Read the model definition and answer for the solid it produces. Units are mm, in the model's axes. A direction names the side the tool comes from. Coordinates: 2 decimals unless noted, no trailing zeros. Loops run counter-clockwise (first coordinate to the right, second up) from the corner with the lowest first, then second, coordinate; pieces in that order, holes last. Notation, with made-up numbers: M 3.5,88.5 L 53.5,88.5 A18 cw 53.5,105.5 Z; hole C 76,38 d10. An arc over 180 degrees is marked long. Put each result on its own line as item: value.
from build123d import *
from build123d.topology import SkipClean

# Parameters (mm, degrees)
SKETCH1_W           = 65
SKETCH1_H           = 18.4
BOSS_EXTRUDE1_DEPTH = 7.5
SKETCH2_R           = 10
BOSS_EXTRUDE2_DEPTH = 7.5
CUT_EXTRUDE1_DEPTH  = 7.5
BOSS_EXTRUDE3_START = -7.5
BOSS_EXTRUDE3_DEPTH = 7.5
CUT_EXTRUDE2_START  = -7.5
CUT_EXTRUDE2_DEPTH  = 7.5
SKETCH6_R           = 2.0193
CUT_EXTRUDE3_DEPTH  = 7.5
SKETCH11_R          = 3.175
CUT_EXTRUDE6_DEPTH  = 81.999212959
SKETCH1_4_W         = 65
SKETCH1_4_H         = 18.4
BOSS_EXTRUDE6_DEPTH = 6.5
CUT_EXTRUDE7_DEPTH  = 81.999212959
SKETCH13_W          = 80
SKETCH13_H          = 33.4
CUT_EXTRUDE8_DEPTH  = 2
SKETCH14_W          = 80
SKETCH14_H          = 33.4
SKETCH14_W_2        = 65
SKETCH14_H_2        = 18.4
BOSS_EXTRUDE7_DEPTH = 2
CUT_EXTRUDE9_DEPTH  = 81.999212959


with BuildPart() as part:
    # Sketch1 → Boss-Extrude1 (new body)
    with BuildSketch(Plane(origin=(0, 0, 0), x_dir=(1, 0, 0), z_dir=(0, 1, 0))):
        Polygon((0, 25.9), (72.5, 25.9), (72.5, -7.5), (-7.5, -7.5), (-7.5, 25.9), align=None)
        with Locations((32.5, 9.2)):
            Rectangle(SKETCH1_W, SKETCH1_H, mode=Mode.SUBTRACT)
    extrude(amount=BOSS_EXTRUDE1_DEPTH)

    # Sketch2 → Boss-Extrude2 (add)
    with BuildSketch(Plane.XY.offset(7.5)):
        with Locations((32.5, 3.75)):
            Circle(SKETCH2_R)
    extrude(amount=-BOSS_EXTRUDE2_DEPTH)

    # Sketch3 → Cut-Extrude1 (cut)
    with BuildSketch(Plane.XY.offset(7.5)):
        with BuildLine():
            ThreePointArc((38.5, 3.75), (33.646103575, 9.639520065), (26.937851135, 6))
            Line((26.937851135, 6), (38.062148865, 1.5))
            ThreePointArc((38.062148865, 1.5), (38.389520065, 2.603896425), (38.5, 3.75))
        make_face()
        with BuildLine():
            Line((38.062148865, 1.5), (26.937851135, 6))
            ThreePointArc((26.937851135, 6), (30.25, -1.812148865), (38.062148865, 1.5))
        make_face()
    extrude(amount=-CUT_EXTRUDE1_DEPTH, mode=Mode.SUBTRACT)

    # Sketch4 → Boss-Extrude3 (add)
    with BuildSketch(Plane(origin=(0, 0, -25.9), x_dir=(-1, 0, 0), z_dir=(0, 0, -1)).offset(BOSS_EXTRUDE3_START)):
        with BuildLine():
            Line((-23.229751891, 0), (-32.5, 0))
            Line((-32.5, 0), (-41.770248109, 0))
            ThreePointArc((-41.770248109, 0), (-32.5, -6.25), (-23.229751891, 0))
        make_face()
        with BuildLine():
            Line((-41.770248109, 7.5), (-32.5, 7.5))
            Line((-32.5, 7.5), (-23.229751891, 7.5))
            ThreePointArc((-23.229751891, 7.5), (-32.5, 13.75), (-41.770248109, 7.5))
        make_face()
        with BuildLine():
            Line((-23.229751891, 7.5), (-32.5, 7.5))
            Line((-32.5, 7.5), (-32.5, 0))
            Line((-32.5, 0), (-23.229751891, 0))
            ThreePointArc((-23.229751891, 0), (-22.684133225, 1.839827375), (-22.5, 3.75))
            ThreePointArc((-22.5, 3.75), (-22.684133225, 5.660172625), (-23.229751891, 7.5))
        make_face()
        with BuildLine():
            Line((-32.5, 0), (-32.5, 7.5))
            Line((-32.5, 7.5), (-41.770248109, 7.5))
            ThreePointArc((-41.770248109, 7.5), (-42.5, 3.75), (-41.770248109, 0))
            Line((-41.770248109, 0), (-32.5, 0))
        make_face()
    extrude(amount=BOSS_EXTRUDE3_DEPTH)

    # Sketch5 → Cut-Extrude2 (cut)
    with BuildSketch(Plane(origin=(0, 0, -25.9), x_dir=(-1, 0, 0), z_dir=(0, 0, -1)).offset(CUT_EXTRUDE2_START)):
        with BuildLine():
            ThreePointArc((-26.5, 3.75), (-31.353896425, 9.639520065), (-38.062148865, 6))
            Line((-38.062148865, 6), (-26.937851135, 1.5))
            ThreePointArc((-26.937851135, 1.5), (-26.610479935, 2.603896425), (-26.5, 3.75))
        make_face()
        with BuildLine():
            Line((-26.937851135, 1.5), (-38.062148865, 6))
            ThreePointArc((-38.062148865, 6), (-34.75, -1.812148865), (-26.937851135, 1.5))
        make_face()
    extrude(amount=CUT_EXTRUDE2_DEPTH, mode=Mode.SUBTRACT)

    # Sketch6 → Cut-Extrude3 (cut)
    with BuildSketch(Plane(origin=(0, 0, -25.9), x_dir=(-1, 0, 0), z_dir=(0, 0, -1))):
        with Locations((-7.1, 3.75)):
            Circle(SKETCH6_R)
        with Locations((-57.9, 3.75)):
            Circle(SKETCH6_R)
    extrude(amount=-CUT_EXTRUDE3_DEPTH, mode=Mode.SUBTRACT)

    # Sketch11 → Cut-Extrude6 (cut, through all)
    with BuildSketch(Plane(origin=(0, 0, -25.9), x_dir=(-1, 0, 0), z_dir=(0, 0, -1))):
        with Locations((-67.5, 3.75)):
            Circle(SKETCH11_R)
    extrude(amount=-CUT_EXTRUDE6_DEPTH, mode=Mode.SUBTRACT)

    # Sketch1_4 → Boss-Extrude6 (add)
    with BuildSketch(Plane(origin=(0, 0, 0), x_dir=(1, 0, 0), z_dir=(0, 1, 0))):
        Polygon((0, 25.9), (72.5, 25.9), (72.5, -7.5), (-7.5, -7.5), (-7.5, 25.9), align=None)
        with Locations((32.5, 9.2)):
            Rectangle(SKETCH1_4_W, SKETCH1_4_H, mode=Mode.SUBTRACT)
    extrude(amount=-BOSS_EXTRUDE6_DEPTH)

    # Sketch3_4 → Cut-Extrude7 (cut, through all)
    with SkipClean():  # the faces are left unmerged after this step: merging them gives an invalid solid
        with BuildSketch(Plane.XY.offset(7.5)):
            with BuildLine():
                ThreePointArc((38.5, 3.75), (33.646103575, 9.639520065), (26.937851135, 6))
                Line((26.937851135, 6), (38.062148865, 1.5))
                ThreePointArc((38.062148865, 1.5), (38.389520065, 2.603896425), (38.5, 3.75))
            make_face()
            with BuildLine():
                Line((38.062148865, 1.5), (26.937851135, 6))
                ThreePointArc((26.937851135, 6), (30.25, -1.812148865), (38.062148865, 1.5))
            make_face()
        extrude(amount=-CUT_EXTRUDE7_DEPTH, mode=Mode.SUBTRACT)

    # Sketch13 → Cut-Extrude8 (cut)
    with SkipClean():  # the faces are left unmerged after this step: merging them gives an invalid solid
        with BuildSketch(Plane.XZ.offset(6.5)):
            with Locations((32.5, -9.2)):
                Rectangle(SKETCH13_W, SKETCH13_H)
        extrude(amount=-CUT_EXTRUDE8_DEPTH, mode=Mode.SUBTRACT)

    # Sketch14 → Boss-Extrude7 (add)
    with SkipClean():  # the faces are left unmerged after this step: merging them gives an invalid solid
        with BuildSketch(Plane(origin=(0, 7.5, 0), x_dir=(1, 0, 0), z_dir=(0, 1, 0))):
            with Locations((32.5, 9.2)):
                Rectangle(SKETCH14_W, SKETCH14_H)
            with Locations((32.5, 9.2)):
                Rectangle(SKETCH14_W_2, SKETCH14_H_2, mode=Mode.SUBTRACT)
        extrude(amount=BOSS_EXTRUDE7_DEPTH)

    # Sketch3_5 → Cut-Extrude9 (cut, through all)
    with SkipClean():  # the faces are left unmerged after this step: merging them gives an invalid solid
        with BuildSketch(Plane.XY.offset(7.5)):
            with BuildLine():
                ThreePointArc((38.5, 3.75), (33.646103575, 9.639520065), (26.937851135, 6))
                Line((26.937851135, 6), (38.062148865, 1.5))
                ThreePointArc((38.062148865, 1.5), (38.389520065, 2.603896425), (38.5, 3.75))
            make_face()
            with BuildLine():
                Line((38.062148865, 1.5), (26.937851135, 6))
                ThreePointArc((26.937851135, 6), (30.25, -1.812148865), (38.062148865, 1.5))
            make_face()
        extrude(amount=-CUT_EXTRUDE9_DEPTH, mode=Mode.SUBTRACT)


solid = part.part
1) Find section B-B, the plane x = 43.5. Write down the section's boundary in (y, z).
Answer list:
outline: M -4.5,-25.9 L 9.5,-25.9 L 9.5,-18.4 L -4.5,-18.4 Z; M -4.5,0 L 9.5,0 L 9.5,7.5 L -4.5,7.5 Z
2) Straight lines are drawn through the part: line 1 (X direction, y = 4, z = 6); line 2 (X direction, y = -2.75, z = -8); line 3 (X direction, y = 1.5, z = -21). For each, find the intervals that lie inside material, in ascending order. Write a range as [from, to].
Answer list:
line 1: x = [-7.5, 26.51], [38.49, 64.33], [70.67, 72.5]
line 2: x = [-7.5, 0], [65, 72.5]
line 3: x = [-7.5, 26.94], [38.06, 65.26], [69.74, 72.5]
3) Find section D-D, the plane y = 11.75. Write down the section's boundary in (x, z), plus the area to 3 significant figures.
Answer list:
outline: M 26.5,-25.9 L 38.5,-25.9 L 38.5,-18.4 L 26.5,-18.4 Z; M 26.5,0 L 38.5,0 L 38.5,7.5 L 26.5,7.5 Z
area: 180 mm^2
4) Given pin 1 Ø4 at (x, z) = (48.5, -19) entering from +Y; pin 2 Ø5 at (x, y) = (67.5, 3.75) entering from +Z, each flat-ended and moving along its own axis, determine where each tip first touches the part or whether it passes through.
Answer list:
pin 1: stops at y = 9.5
pin 2: passes through
5) Determine the mould class of faces 6 (the cylindrical face through (32.63, 13.75, 3.8)), 7 (the cylindrical face through (5.235, 2.977, -22.202)), 8 (the flat face through (65, -1, -9)) for opening direction Y: released by +Y, released by -Y, zero draft, split by the parting line, or undercut.
Answer list:
face 6: released by +Y
face 7: undercut
face 8: zero draft
6) Find section C-C, the plane z = -16. Write down the section's boundary in (x, y) (3 decimals).
Answer list:
outline: M -7.5,-4.5 L 0,-4.5 L 0,9.5 L -7.5,9.5 Z; M 65,-4.5 L 72.5,-4.5 L 72.5,9.5 L 65,9.5 L 65,5.707 A3.175 cw long 65,1.793 Z
7) Which of the six approach directions +Z, -Z, +X, -X, +Y, -Y give full straight-line access (tool end or side, diameter ignored) to faces 1 (the flat face through (67, 9.5, -9)), 2 (the flat face through (32, -4.5, -20)), 3 (the flat face through (-2, 9.5, -9)), 4 (the cylindrical face through (59.917, 3.839, -22.202)), 5 (the cylindrical face through (32.37, 13.75, -22.1))?
Answer list:
face 1: +Z, -Z, +X, +Y
face 2: +Z, -Z, +X, -X, -Y
face 3: +Z, -Z, -X, +Y
face 4: -Z
face 5: +Z, -Z, +Y
8) Find section A-A, the plane x = 57.9. Write down the section's boundary in (y, z), plus the area to 3 significant figures.
Answer list:
outline: M -4.5,-25.9 L 1.73,-25.9 L 1.73,-18.4 L -4.5,-18.4 Z; M -4.5,0 L 9.5,0 L 9.5,7.5 L -4.5,7.5 Z; M 5.77,-25.9 L 9.5,-25.9 L 9.5,-18.4 L 5.77,-18.4 Z
area: 180 mm^2
